Can you work these out from the drawing? Everything is in mm from the part's minimum corner. A direction names the side the tool comes from. Round coordinates to 2 decimals unless told otherwise and drop trailing zeros. One line per question, with ' | ' between items. Start each with the question number.
1. Thinking about a two-plate mould opening in Y: for the marked faces 1, 2 and 3, which applies, released by +Y, released by -Y, zero draft, split by the parting line, or undercut?
2. If I drill on line 1 along X through (y, z) = (57, 39.5) (1 decimal); line 2 along Y through (x, z) = (6.75, 21.5) (1 decimal); line 3 along Z through (x, y) = (6, 16) (1 decimal), over which ranges is the centre line in solid material (lowest first)? Write a range as [from, to].
3. For pin 1 Ø15.5 at (y, z) = (22.19, 22.19) entering from -X (1 decimal); pin 2 Ø4 at (x, y) = (12, 15) entering from -Z; pin 3 Ø8.5 at (y, z) = (60.36, 22.19) entering from +X; pin 4 Ø1 at (x, y) = (7.5, 34) entering from +Z, each with a flat end and sliding along its axis, tell me the tip position at first contact or that it passes through.
4. For the marked faces 4 and 5, which set-ups out of +Z, -Z, +X, -X, +Y, -Y let a thin tool reach every point of the face, with its end or its side?
5. Imagine slicing it at C-C, the plane y = 20.5. State how many separate pieces and enclosed holes the cut face has, and give its area (3 significant figures).
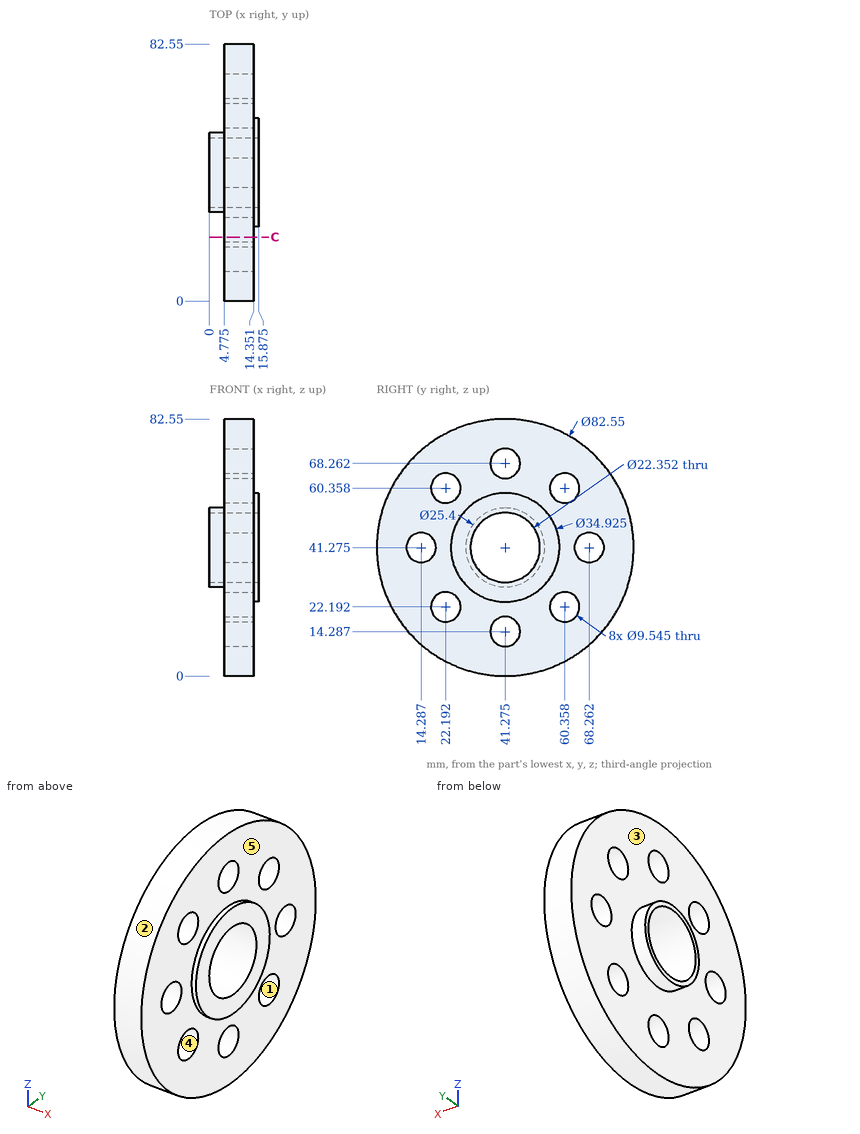
Geometry results:
1) face 1: undercut | face 2: split by the parting line | face 3: zero draft
2) line 1: x = [4.8, 15.9] | line 2: y = [5, 17.5], [26.9, 55.6], [65.1, 77.5] | line 3: z = [8.6, 36.8], [45.7, 73.9]
3) pin 1: stops at x = 4.8 | pin 2: stops at z = 7.89 | pin 3: passes through | pin 4: stops at z = 81.99
4) face 4: +X, -X | face 5: +X
5) separate pieces: 3 | enclosed holes: 0 | area: 512 mm2
